Verification items for the finished model (mm, model axes). A direction names the side the tool comes from. Coordinates: 2 decimals unless noted, no trailing zeros. Order: outer loops, then holes, each group sorted by start corner. A loop starts at its lowest first (then second) coordinate and runs counter-clockwise, first axis right, second up.
Q1. Depth check by flat-ended pin: P1, Ø2.5, axis at y = 1.1, z = -18.72, coming from the +X side; P2, Ø14.5, axis at y = -7.86, z = 14.57, coming from the +X side; P3, Ø5, axis at x = 6.35, z = 0, coming from the -Y side. Enter the tip coordinate at first touch or a pass-through.
Q2. Draft check along Y on faces 1 (the conical face through (6.65, 1.58, -63.04)), 2 (the cylindrical face through (4.643, -18.783, -60.823)), 3 (the flat face through (7.62, -1, -19)). Enter one of: pulls with the +Y half, pulls with the -Y half, needs draft (parallel to the pull), parting line crosses it, or undercut.
Q3. Cross-section at C-C, the plane x = 11. Count the separate pieces of the cut face and the enclosed holes in it, and give its area (3 significant figures).
Q4. Cross-section at B-B, the plane z = 38.1. Record the boundary of the cut face in (x, y), and give its area (3 significant figures).
Q5. Set-up check for faces 4 (the cylindrical face through (6.4, -13.7, 47.4)), 5 (the cylindrical face through (10.196, -9.525, -59.338)), 6 (the cylindrical face through (7.04, -18.78, 54.05)): record each of +Z, -Z, +X, -X, +Y, -Y from which the full face is reachable in a straight line by a thin tool's end or side.
Q6. Cross-section at A-A, the plane y = -22. Record the boundary of the cut face in (x, z) (3 decimals).
Q7. Thickness scan on line 1 (Y direction, x = 2.25, z = 38.1); line 2 (Z direction, x = 6.35, y = -23.5) (3 decimals); line 3 (Z direction, x = 12, y = -5). Record the ranges inside material, lowest first.
from build123d import *

# Parameters (mm, degrees)
SKETCH1_R                       = 1.5875
BOSS_EXTRUDE1_DEPTH             = 12.7
SKETCH2_R                       = 7.9375
CUT_EXTRUDE1_DEPTH              = 5.08
F_1_4_0_25_DIAMETER_HOLE1_D     = 6.35
F_1_4_0_25_DIAMETER_HOLE1_DEPTH = 38.1
F_1_4_0_25_DIAMETER_HOLE1_TIP   = 1.907732465
CUT_EXTRUDE2_DEPTH              = 25.4


with BuildPart() as part:
    # Sketch1 → Boss-Extrude1 (new body)
    # profile 1 of 2: a face of its own
    with BuildSketch(Plane(origin=(0, 0, 0), x_dir=(0, 0, -1), z_dir=(1, 0, 0))):
        with BuildLine():
            Line((-76.2, 38.1), (-76.2, 0))
            Line((-76.2, 0), (-39.6875, 0))
            ThreePointArc((-39.6875, 0), (-38.1, 1.5875), (-36.5125, 0))
            Line((-36.5125, 0), (17.574154238, 0))
            ThreePointArc((17.574154238, 0), (18.13214729, 2.569713286), (20.31003158, 1.096077429))
            ThreePointArc((20.31003158, 1.096077429), (20.196167438, 0.505693139), (19.870908922, 0))
            Line((19.870908922, 0), (76.2, 0))
            Line((76.2, 0), (76.2, 38.1))
            Line((76.2, 38.1), (-76.2, 38.1))
        make_face()
    # profile 2 of 2: a face of its own
    with BuildSketch(Plane(origin=(0, 0, 0), x_dir=(0, 0, -1), z_dir=(1, 0, 0))):
        with BuildLine():
            Line((-39.6875, 0), (-76.2, 0))
            Line((-76.2, 0), (-76.2, -38.1))
            Line((-76.2, -38.1), (76.2, -38.1))
            Line((76.2, -38.1), (76.2, 0))
            Line((76.2, 0), (19.870908922, 0))
            ThreePointArc((19.870908922, 0), (18.72253158, -0.491422571), (17.574154238, 0))
            Line((17.574154238, 0), (-36.5125, 0))
            ThreePointArc((-36.5125, 0), (-38.1, -1.5875), (-39.6875, 0))
        make_face()
        with Locations((-14.571224015, -7.860160654)):
            Circle(SKETCH1_R, mode=Mode.SUBTRACT)
        with Locations((51.408255992, -9.873506971)):
            Circle(SKETCH1_R, mode=Mode.SUBTRACT)
    extrude(amount=BOSS_EXTRUDE1_DEPTH)

    # Sketch2 → Cut-Extrude1 (cut)
    with BuildSketch(Plane.ZY.offset(-12.7)):
        with Locations((38.1, 0)):
            Circle(SKETCH2_R)
        with Locations((14.571224015, -7.860160654)):
            Circle(SKETCH2_R)
        with Locations((-18.72253158, 1.096077429)):
            Circle(SKETCH2_R)
        with Locations((-51.408255992, -9.873506971)):
            Circle(SKETCH2_R)
    extrude(amount=CUT_EXTRUDE1_DEPTH, mode=Mode.SUBTRACT)

    # 1_4 _0.25_ Diameter Hole1
    with Locations(Plane.XZ.offset(38.1)):
        with Locations((6.35, -63.5), (6.35, 0), (6.35, 57.15)):
            Hole(F_1_4_0_25_DIAMETER_HOLE1_D / 2, depth=F_1_4_0_25_DIAMETER_HOLE1_DEPTH)
            with Locations((0, 0, -(F_1_4_0_25_DIAMETER_HOLE1_DEPTH + F_1_4_0_25_DIAMETER_HOLE1_TIP / 2))):  # 118° drill point
                Cone(0, F_1_4_0_25_DIAMETER_HOLE1_D / 2, F_1_4_0_25_DIAMETER_HOLE1_TIP, mode=Mode.SUBTRACT)

    # Sketch5 → Cut-Extrude2 (cut)
    with BuildSketch(Plane(origin=(12.7, 0, 0), x_dir=(0, 0, -1), z_dir=(1, 0, 0))):
        with BuildLine():
            Line((-45.085, -12.7), (-26.035, -12.7))
            ThreePointArc((-26.035, -12.7), (-23.78993597, -13.62993597), (-22.86, -15.875))
            Line((-22.86, -15.875), (-22.86, -28.575))
            ThreePointArc((-22.86, -28.575), (-23.78993597, -30.82006403), (-26.035, -31.75))
            Line((-26.035, -31.75), (-45.085, -31.75))
            ThreePointArc((-45.085, -31.75), (-47.33006403, -30.82006403), (-48.26, -28.575))
            Line((-48.26, -28.575), (-48.26, -15.875))
            ThreePointArc((-48.26, -15.875), (-47.33006403, -13.62993597), (-45.085, -12.7))
        make_face()
    extrude(amount=-CUT_EXTRUDE2_DEPTH, mode=Mode.SUBTRACT)


solid = part.part
Check values:
1. P1: passes through
1. P2: stops at x = 7.62
1. P3: stops at y = 0.41
2. face 1: pulls with the -Y half
2. face 2: needs draft
2. face 3: undercut
3. separate pieces: 1
3. enclosed holes: 5
3. area: 10,300 mm2
4. outline: (0, -38.1) - (12.7, -38.1) - (12.7, -31.75) - (0, -31.75) - close; (0, -12.7) - (12.7, -12.7) - (12.7, -7.94) - (7.62, -7.94) - (7.62, -1.59) - (0, -1.59) - close; (0, 1.59) - (7.62, 1.59) - (7.62, 7.94) - (12.7, 7.94) - (12.7, 38.1) - (0, 38.1) - close
4. area: 621 mm2
5. face 4: +X, -X
5. face 5: +X
5. face 6: -Y
6. outline: (0, -76.2) - (12.7, -76.2) - (12.7, 22.86) - (0, 22.86) - close; (0, 48.26) - (12.7, 48.26) - (12.7, 76.2) - (0, 76.2) - close; hole circle Ø6.35 at (6.35, -63.5); hole circle Ø6.35 at (6.35, 0); hole circle Ø6.35 at (6.35, 57.15)
7. line 1: y = -38.1 to -31.75, -12.7 to -1.59, 1.59 to 38.1
7. line 2: z = -76.2 to -66.675, -60.325 to -3.175, 3.175 to 22.86, 48.26 to 53.975, 60.325 to 76.2
7. line 3: z = -76.2 to -57.67, -45.14 to -23.81, -13.64 to 7.17, 21.98 to 31.94, 44.26 to 76.2
